For this review, take the finished solid that the model builds, in its own axes (mm). Face numbers are marked on the shaded views. Give positions to 0.01 mm unless a question says otherwise; leave off trailing zeros. Write each loop counter-clockwise with the first axis right and the second up, starting at its lowest first coordinate (ties: lowest second). Pieces come first, ordered by that corner, then holes.
Q1. Insertion check: P1, Ø1, axis at y = -32.5, z = 5, coming from the -X side; P2, Ø12, axis at x = 0, y = 25.93, coming from the +Z side. Each pin has a flat end and moves straight along its axis. Give the tip position at first contact, or say it passes through.
Q2. We need section D-D (x = 34). Write out the cut boundary in (y, z).
Q3. We need section A-A (x = 0). Write out the cut boundary in (y, z).
Q4. We need section B-B (y = 0). Write out the cut boundary in (x, z).
Q5. We need section C-C (y = 30). Write out the cut boundary in (x, z).
Q6. For line 1 (Y direction, x = 0, z = 3.5); line 2 (Y direction, x = 2, z = 4.75); line 3 (X direction, y = 3.5, z = 3.5), list the stretches that pass through material, from the lowest coordinate up.
Q7. Mouldability with a two-part tool opening along X and no side actions: class the marked faces 1, 2, 3 and 4 as released by +X, released by -X, zero draft, split by the parting line, or undercut.
```python
from build123d import *

# Parameters (mm, degrees)
F0_R     = 50
F2_DEPTH = 10
F4_D     = 15
F6_D     = 15


with BuildPart() as f2:
    # F0 (on Top) → F2 (new body)
    with BuildSketch(Plane.XY):
        Circle(F0_R)
    extrude(amount=F2_DEPTH)

    # F4 (through all)
    with Locations(Plane.XY.offset(10)):
        with Locations((0, 25.931375)):
            Hole(F4_D / 2)

    # F6 (through all)
    with Locations(Plane(origin=(0, 0, 0), x_dir=(1, 0, 0), z_dir=(0, 0, -1))):
        with Locations((0, 0)):
            Hole(F6_D / 2)


solid = f2.part
```
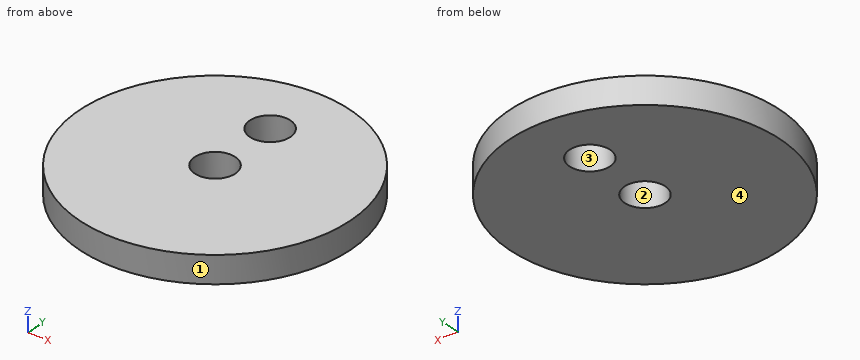
Computed:
1. P1: stops at x = -38.42
1. P2: passes through
2. outline: (-36.66, 0) - (36.66, 0) - (36.66, 10) - (-36.66, 10) - close
3. outline: (-50, 0) - (-7.5, 0) - (-7.5, 10) - (-50, 10) - close; (7.5, 0) - (18.43, 0) - (18.43, 10) - (7.5, 10) - close; (33.43, 0) - (50, 0) - (50, 10) - (33.43, 10) - close
4. outline: (-50, 0) - (-7.5, 0) - (-7.5, 10) - (-50, 10) - close; (7.5, 0) - (50, 0) - (50, 10) - (7.5, 10) - close
5. outline: (-40, 0) - (-6.3, 0) - (-6.3, 10) - (-40, 10) - close; (6.3, 0) - (40, 0) - (40, 10) - (6.3, 10) - close
6. line 1: y = -50 to -7.5, 7.5 to 18.43, 33.43 to 50
6. line 2: y = -49.96 to -7.23, 7.23 to 18.7, 33.16 to 49.96
6. line 3: x = -49.88 to -6.63, 6.63 to 49.88
7. face 1: split by the parting line
7. face 2: undercut
7. face 3: undercut
7. face 4: zero draft
